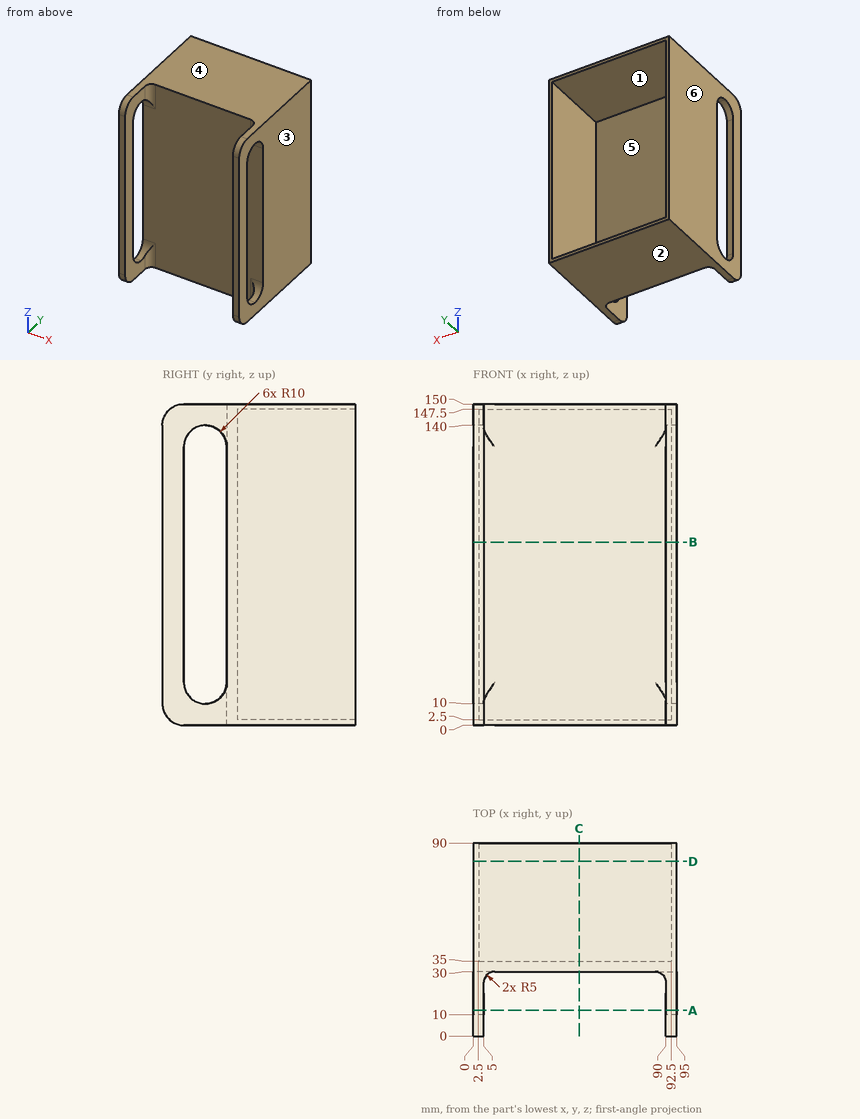
Job drawing, mm, ordinate dimensions from the low corner. One solid piece. A direction names the side the tool comes from. Round coordinates to 2 decimals unless told otherwise and drop trailing zeros. Loops run counter-clockwise (first coordinate to the right, second up) from the corner with the lowest first, then second, coordinate; pieces in that order, holes last.
Item 1: 3-axis set-ups, long thin cutter, end or side, ignore diameter. For the marked faces 5 and 6: which of +Z, -Z, +X, -X, +Y, -Y reach the whole face in a straight line?
Item 2: Cut at C-C, the plane x = 49.5. Give the cut face in (y, z), then the cut area to 4 significant figures.
Item 3: Mould opens along Z. For the marked faces 1, 2, 3 and 4 say: +Z half, -Z half, draft (parallel to the pull), parting line (faces both ways), or undercut.
Item 4: Cut at B-B, the plane z = 85.5. Give the cut face in (x, y).
Item 5: Drill centre lines: line 1 (Z direction, x = 61, y = 37); line 2 (X direction, y = 48, z = 114); line 3 (Y direction, x = 76.5, z = 71). Where is each one in solid material? Low to high.
Item 6: Cut at A-A, the plane y = 12. Give the cut face in (x, z), then the cut area to 3 significant figures.
Item 7: Drop flat-ended pins along their axis: P1, Ø4, axis at x = 85, z = 104.5, coming from the +Y side; P2, Ø8, axis at x = 53.5, z = 60.5, coming from the -Y side. Give the stop position or say it passes through.
Item 8: Cut at D-D, the plane y = 81.5. Give the cut face in (x, z), then the cut area to 3 significant figures.
A:
1. face 5: +Y
1. face 6: +Z, -Z, -X, +Y, -Y
2. outline: (30, 0) - (90, 0) - (90, 2.5) - (35, 2.5) - (35, 147.5) - (90, 147.5) - (90, 150) - (30, 150) - close
2. area: 1,025 mm2
3. face 1: undercut
3. face 2: -Z half
3. face 3: draft
3. face 4: +Z half
4. outline: (0, 0) - (5, 0) - (5, 10) - (0, 10) - close; (0, 30) - (95, 30) - (95, 90) - (92.5, 90) - (92.5, 35) - (2.5, 35) - (2.5, 90) - (0, 90) - close; (90, 0) - (95, 0) - (95, 10) - (90, 10) - close
5. line 1: z = 0 to 2.5, 147.5 to 150
5. line 2: x = 0 to 2.5, 92.5 to 95
5. line 3: y = 30 to 35
6. outline: (0, 0) - (5, 0) - (5, 14) - (0, 14) - close; (0, 136) - (5, 136) - (5, 150) - (0, 150) - close; (90, 0) - (95, 0) - (95, 14) - (90, 14) - close; (90, 136) - (95, 136) - (95, 150) - (90, 150) - close
6. area: 280 mm2
7. P1: stops at y = 35
7. P2: stops at y = 30
8. outline: (0, 0) - (95, 0) - (95, 150) - (0, 150) - close; hole (2.5, 2.5) - (92.5, 2.5) - (92.5, 147.5) - (2.5, 147.5) - close
8. area: 1,200 mm2
